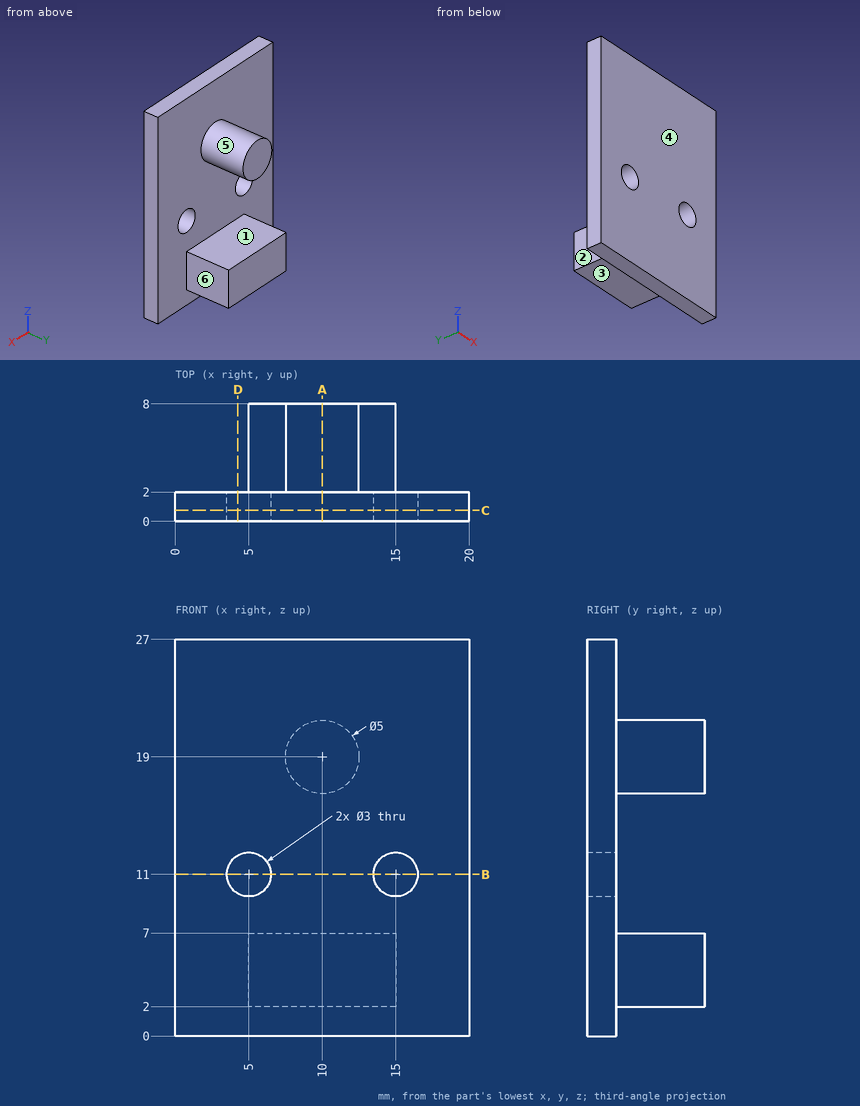
Part print with two shaded views. Sizes in mm from the minimum x, y, z corner. A direction names the side the tool comes from. Coordinates: 2 decimals unless noted, no trailing zeros. Write each loop counter-clockwise with the first axis right and the second up, starting at its lowest first coordinate (ties: lowest second). Pieces come first, ordered by that corner, then holes.
(1) Cut at D-D on x = 4.25. List the corners of the cut face in (y, z).
(2) 3-axis set-ups, long thin cutter, end or side, ignore diameter. For the marked faces 4, 5 and 6: which of +Z, -Z, +X, -X, +Y, -Y reach the whole face in a straight line?
(3) Drill centre lines: line 1 (X direction, y = 1.2, z = 11); line 2 (Z direction, x = 15, y = 0.6); line 3 (Y direction, x = 17.75, z = 12). Where is each one in solid material? Low to high.
(4) Cut at A-A on x = 10. List the corners of the cut face in (y, z), and give its area (3 significant figures).
(5) Cut at C-C on y = 0.75. List the corners of the cut face in (x, z), and give its area (3 significant figures).
(6) Pin check, flat tips, straight feed: pin 1 Ø3 at (x, y) = (11, 5.5) entering from +Z; pin 2 Ø5 at (x, z) = (15, 11) entering from +Y; pin 3 Ø4 at (y, z) = (6, 4.5) entering from +X. Stop position of each tip, or through.
(7) Cut at B-B on z = 11. List the corners of the cut face in (x, y).
(8) Mould opens along Z. For the marked faces 1, 2 and 3 say: pulls with the +Z half, pulls with the -Z half, needs draft (parallel to the pull), parting line crosses it, or undercut.
Working result:
1. outline: (0, 0) - (2, 0) - (2, 9.7) - (0, 9.7) - close; (0, 12.3) - (2, 12.3) - (2, 27) - (0, 27) - close
2. face 4: +Z, -Z, +X, -X, -Y
2. face 5: +Y
2. face 6: +Z, -Z, +X, +Y
3. line 1: x = 0 to 3.5, 6.5 to 13.5, 16.5 to 20
3. line 2: z = 0 to 9.5, 12.5 to 27
3. line 3: y = 0 to 2
4. outline: (0, 0) - (2, 0) - (2, 2) - (8, 2) - (8, 7) - (2, 7) - (2, 16.5) - (8, 16.5) - (8, 21.5) - (2, 21.5) - (2, 27) - (0, 27) - close
4. area: 114 mm2
5. outline: (0, 0) - (20, 0) - (20, 27) - (0, 27) - close; hole circle Ø3 at (5, 11); hole circle Ø3 at (15, 11)
5. area: 526 mm2
6. pin 1: stops at z = 21.5
6. pin 2: stops at y = 2
6. pin 3: stops at x = 15
7. outline: (0, 0) - (3.5, 0) - (3.5, 2) - (0, 2) - close; (6.5, 0) - (13.5, 0) - (13.5, 2) - (6.5, 2) - close; (16.5, 0) - (20, 0) - (20, 2) - (16.5, 2) - close
8. face 1: undercut
8. face 2: needs draft
8. face 3: pulls with the -Z half
